from build123d import *
from OCP.BRepFilletAPI import BRepFilletAPI_MakeChamfer

# Parameters (mm, degrees)
BOSS_EXTRUDE1_START = -0.7874
SKETCH3_R           = 19.05
SKETCH3_R_2         = 9.525
BOSS_EXTRUDE1_DEPTH = 3.175
CHAMFER1_SIZE       = 0.15748
CHAMFER1_SIZE2      = 0.09092112
FILLET1_R           = 0.47244


with BuildPart() as part:
    # Sketch3 → Boss-Extrude1 (new body)
    with BuildSketch(Plane.XY.offset(BOSS_EXTRUDE1_START)):
        Circle(SKETCH3_R)
        Circle(SKETCH3_R_2, mode=Mode.SUBTRACT)
    extrude(amount=BOSS_EXTRUDE1_DEPTH)

    # Chamfer1: one chamfer whose edges measure the first distance from different faces: ONE call of the kernel's chamfer builder (chamfer() names one face for all edges)
    chamfer1_edges_1 = [part.edges().sort_by_distance(p)[0] for p in [
        (-19.05, 0, 2.3876),
    ]]
    chamfer1_side_1 = [part.faces().sort_by_distance(p)[0] for p in [
        (-19.05, 0, 0.8001),
    ]]
    chamfer1_edges_2 = [part.edges().sort_by_distance(p)[0] for p in [
        (-9.525, 0, 2.3876),
    ]]
    chamfer1_side_2 = [part.faces().sort_by_distance(p)[0] for p in [
        (-9.525, 0, 0.8001),
    ]]
    chamfer1 = BRepFilletAPI_MakeChamfer(part.part.solid().wrapped)
    for e in chamfer1_edges_1:
        chamfer1.Add(CHAMFER1_SIZE, CHAMFER1_SIZE2, e.wrapped, chamfer1_side_1[0].wrapped)  # the first distance lies on this face
    for e in chamfer1_edges_2:
        chamfer1.Add(CHAMFER1_SIZE, CHAMFER1_SIZE2, e.wrapped, chamfer1_side_2[0].wrapped)  # the first distance lies on this face
    add(Compound.cast(chamfer1.Shape()), mode=Mode.REPLACE)

    # Fillet1
    # the kernel refuses this fillet: 0.47244 mm, written as the material it takes off along each edge
    with BuildSketch(Plane(origin=(0, 0, 2.3876), x_dir=(1, 0, 0), z_dir=(0, -1, 0))) as fillet1_piece_1:
        with BuildLine():
            CenterArc((18.697864015, -0.47244), FILLET1_R, 41.810314896, 48.189685104)
            Line((18.697864015, 0), (18.697864015, 0.0094488))
            Line((18.697864015, 0.0094488), (18.95907888, 0.0094488))
            Line((18.95907888, 0.0094488), (18.96726178, 0.0047244))
            ThreePointArc((18.96726178, 0.0047244), (19.012722341, -0.0740156), (19.05704272, -0.1511808))
            Line((19.05704272, -0.1511808), (19.05, -0.15748))
        make_face()
    revolve(axis=Axis((0, 0, 2.3876), (0, 0, 1)), mode=Mode.SUBTRACT)
    with BuildSketch(Plane(origin=(0, 0, 2.3876), x_dir=(1, 0, 0), z_dir=(0, -1, 0))) as fillet1_piece_2:
        with BuildLine():
            CenterArc((9.877135985, -0.47244), FILLET1_R, 90, 48.189685104)
            Line((9.525, -0.15748), (9.51795728, -0.1511808))
            ThreePointArc((9.51795728, -0.1511808), (9.562277659, -0.0740156), (9.60773822, 0.0047244))
            Line((9.60773822, 0.0047244), (9.61592112, 0.0094488))
            Line((9.61592112, 0.0094488), (9.877135985, 0.0094488))
            Line((9.877135985, 0.0094488), (9.877135985, 0))
        make_face()
    revolve(axis=Axis((0, 0, 2.3876), (0, 0, 1)), mode=Mode.SUBTRACT)


solid = part.part
Check sheet for the modelled part. Datum: model origin and axes. Units: mm. Round coordinates to 2 decimals unless told otherwise and drop trailing zeros. Loops run counter-clockwise (first coordinate to the right, second up) from the corner with the lowest first, then second, coordinate; pieces in that order, holes last. Notation, with made-up numbers: M -24.5,-0.5 L 15.5,-0.5 A17 ccw 15.5,32.5 Z; hole C 24.25,54 d10. An arc over 180 degrees is marked long. One line per question, with ' | ' between items. Start each with the question number.
Item 1: Scan lines: probe 1 along Y at (x, z) = (0, 1.15) (3 decimals); probe 2 along X at (y, z) = (7.5, 1.6); probe 3 along Y at (x, z) = (-3, -0.5). Record each from-to range of solid material in increasing order.
Item 2: Gauge pin test, flat end, axial feed: pin 1 Ø1.5 at (y, z) = (-11.5, 0) entering from +X. Record the tip position at first contact, or that the pin passes through.
Item 3: Section check A-A (y = 0). Record the boundary of the cut face in (x, z) (3 decimals), and give its area (3 significant figures).
Item 4: Section check C-C (z = 0.95). Record the boundary of the cut face in (x, y) (3 decimals), and give its area (3 significant figures).
Item 5: Release check for a two-part mould opening along Y. For faces 1 (the face through (-7.559, -5.796, 0.7)), 2 (the face through (-15.12, -11.59, 0.7)), 3 (the face through (8, -8, 2.388)) record: released by +Y, released by -Y, zero draft, split by the parting line, or undercut.
Worked out:
1) probe 1: -19.05 to -9.525, 9.525 to 19.05 | probe 2: -17.51 to -5.87, 5.87 to 17.51 | probe 3: -18.81 to -9.04, 9.04 to 18.81
2) pin 1: x = 15.73
3) outline: M -19.05,-0.787 L -9.525,-0.787 L -9.525,2.23 A0.472 ccw -9.877,2.388 L -18.698,2.388 A0.472 ccw -19.05,2.23 Z; M 9.525,-0.787 L 19.05,-0.787 L 19.05,2.23 A0.472 ccw 18.698,2.388 L 9.877,2.388 A0.472 ccw 9.525,2.23 Z | area: 60.4 mm^2
4) outline: C 0,0 d38.1; hole C 0,0 d19.05 | area: 855 mm^2
5) face 1: undercut | face 2: split by the parting line | face 3: zero draft
